from build123d import *

# Parameters (mm, degrees)
F0_R     = 11
F1_DEPTH = 20
F2_SIZE  = 5
F3_DEPTH = 6
F4_T     = -0.7
F5_W     = 4
F5_H     = 2
F6_DEPTH = 12.5
F7_R     = 0.99999
F8_R     = 0.5
F9_R     = 1


# Not quite as in the source:
# - a fillet or chamfer is up to 0.001 mm smaller than in the source, because OpenCascade refuses the exact size


with BuildPart() as f1:
    # F0 (on Top) → F1 (new body)
    with BuildSketch(Plane.XY):
        Circle(F0_R)
    extrude(amount=F1_DEPTH)

    # F2
    f2_edges = [f1.edges().sort_by_distance(p)[0] for p in [
        (-11, 0, 20),
    ]]
    chamfer(f2_edges, length=F2_SIZE)

    # F3 (add): a face of the model
    f3_faces = [f1.faces().sort_by_distance(p)[0] for p in [
        (0, 0, 20),
    ]]
    extrude(f3_faces, amount=F3_DEPTH)

    # F4
    f4_openings = [f1.faces().sort_by_distance(p)[0] for p in [
        (0, 0, 26),
        (0, 0, 0),
    ]]
    offset(amount=F4_T, openings=f4_openings, kind=Kind.INTERSECTION)

    # F5 (on Front) → F6 (cut, symmetric)
    with BuildSketch(Plane.XZ):
        with Locations((0, 8)):
            Rectangle(F5_W, F5_H)
    extrude(amount=F6_DEPTH, both=True, mode=Mode.SUBTRACT)

    # F7 (radius 1 in the source; OpenCascade refuses exactly that, so slightly less here)
    f7_edges = [f1.edges().sort_by_distance(p)[0] for p in [
        (-2, 10.460307, 7),
        (-2, -10.460307, 7),
        (2, 10.460307, 9),
        (2, -10.460307, 9),
        (-2, 10.460307, 9),
        (-2, -10.460307, 9),
        (2, 10.460307, 7),
        (2, -10.460307, 7),
    ]]
    fillet(f7_edges, radius=F7_R)

    # F8
    f8_edges = [f1.edges().sort_by_distance(p)[0] for p in [
        (-6, 0, 26),
    ]]
    fillet(f8_edges, radius=F8_R)

    # F9
    f9_edges = [f1.edges().sort_by_distance(p)[0] for p in [
        (-11, 0, 15),
    ]]
    fillet(f9_edges, radius=F9_R)


solid = f1.part
Verification items for the finished model (mm, model axes). A direction names the side the tool comes from. Give positions to 0.01 mm unless a question says otherwise; leave off trailing zeros. Order: outer loops, then holes, each group sorted by start corner. A loop starts at its lowest first (then second) coordinate and runs counter-clockwise, first axis right, second up. Notation, with made-up numbers: M 36.25,25 L 69.25,25 A24 cw 69.25,57 Z; hole C 69,54.5 d2. An arc over 180 degrees is marked long. Answer as a JSON object with one key per item and string values. Group by question number.
1) Access from +Z, -Z, +X, -X, +Y, -Y to the whole of each face (thin tool, end or side, straight path). Record for faces 1 (the face through (-6, 0, 23)), 2 (the face through (-2.233, -10.055, 7.252)), 3 (the face through (-1.699, -10.535, 7.285)), 4 (the face through (4.896, -2.03, 22.811)).
2) Scan lines: line 1 along Y through (x, z) = (0, 23.25); line 2 along Y through (x, z) = (0, 4). Record each from-to range of solid material in increasing order. Write a range as [from, to].
3) Depth check by flat-ended pin: pin 1 Ø10 at (x, z) = (7, 20.5) entering from +Y; pin 2 Ø8 at (y, z) = (6, 8.5) entering from +X; pin 3 Ø5 at (y, z) = (1, 19) entering from -X. Enter the tip coordinate at first touch or a pass-through.
4) Mould release check, pull along X, two halves, no side actions. Record for faces 5 (the face through (-1.715, 10.535, 8.699)), 6 (the face through (5.076, -9.759, 7.191)): released by +X, released by -X, zero draft, split by the parting line, or undercut.
5) Cross-section at C-C (z = 6.25). Enter the section's corners in (x, y).
6) Cross-section at B-B (z = 24). Enter the section's corners in (x, y), then the cut area to 4 significant figures.
7) Cross-section at A-A (x = 0). Give the number of separate pieces and of enclosed holes in the cut face, then the cut area to 3 significant figures.
Result sheet:
{
 "1": {"face 1": "+Z", "face 2": "-Z", "face 3": "+Y, -Y", "face 4": "+Z, -Z"},
 "2": {"line 1": "y = [-6, -5.3], [5.3, 6]", "line 2": "y = [-11, -10.3], [10.3, 11]"},
 "3": {"pin 1": "stops at y = 8.76", "pin 2": "stops at x = 10.82", "pin 3": "stops at x = -9.46"},
 "4": {"face 5": "undercut", "face 6": "split by the parting line"},
 "5": {"outline": "C 0,0 d22; hole C 0,0 d20.6"},
 "6": {"outline": "C 0,0 d12; hole C 0,0 d10.6", "area": "24.85 mm2"},
 "7": {"separate pieces": "4", "enclosed holes": "0", "area": "36.3 mm2"}
}
